```python
from build123d import *

# Parameters (mm, degrees)
SKETCH_2_W          = 24
SKETCH_2_H          = 28
EXTRUDE_1_DEPTH     = 22
SKETCH_3_W          = 20
SKETCH_3_H          = 24
CUT_EXTRUDE_1_DEPTH = 18
SKETCH_4_W          = 16
SKETCH_4_H          = 13
CUT_EXTRUDE_3_DEPTH = 26.768197453
SKETCH_6_W          = 20
SKETCH_6_H          = 24
CUT_EXTRUDE_4_DEPTH = 5
SKETCH_7_W          = 24
SKETCH_7_H          = 2
EXTRUDE_3_DEPTH     = 10
SKETCH_8_W          = 24
SKETCH_8_H          = 2
EXTRUDE_4_DEPTH     = 10
EXTRUDE_5_DEPTH     = 35
SKETCH_10_W         = 22
SKETCH_10_H         = 2
EXTRUDE_6_DEPTH     = 25
FILLET_2_R          = 5
SKETCH_11_W         = 7
SKETCH_11_H         = 10
CUT_EXTRUDE_5_DEPTH = 67.80007485
FILLET_4_R          = 2
SKETCH_12_W         = 20
SKETCH_12_H         = 13.5
EXTRUDE_7_DEPTH     = 8
RIB_1_REACH         = 64.944
SKETCH_14_W         = 22
SKETCH_14_H         = 5.5
EXTRUDE_8_DEPTH     = 45
FILLET_5_R          = 2


with BuildPart() as part:
    # ｽｹｯﾁ2 → ﾎﾞｽ - 押し出し1 (new body)
    with BuildSketch(Plane.XY):
        Rectangle(SKETCH_2_W, SKETCH_2_H)
    extrude(amount=EXTRUDE_1_DEPTH)

    # ｽｹｯﾁ3 → ｶｯﾄ - 押し出し1 (cut)
    with BuildSketch(Plane.XY.offset(22)):
        Rectangle(SKETCH_3_W, SKETCH_3_H)
    extrude(amount=-CUT_EXTRUDE_1_DEPTH, mode=Mode.SUBTRACT)

    # ｽｹｯﾁ4 → ｶｯﾄ - 押し出し3 (cut, through all)
    with BuildSketch(Plane.XY.offset(4)):
        with Locations((-4, 0)):
            Rectangle(SKETCH_4_W, SKETCH_4_H)
    extrude(amount=-CUT_EXTRUDE_3_DEPTH, mode=Mode.SUBTRACT)

    # ｽｹｯﾁ6 → ｶｯﾄ - 押し出し4 (cut)
    with BuildSketch(Plane.ZY.offset(12)):
        with Locations((12, 0)):
            Rectangle(SKETCH_6_W, SKETCH_6_H)
    extrude(amount=-CUT_EXTRUDE_4_DEPTH, mode=Mode.SUBTRACT)

    # ｽｹｯﾁ7 → ﾎﾞｽ - 押し出し3 (add)
    with BuildSketch(Plane.XZ.offset(14)):
        with Locations((0, 1)):
            Rectangle(SKETCH_7_W, SKETCH_7_H)
    extrude(amount=EXTRUDE_3_DEPTH)

    # ｽｹｯﾁ8 → ﾎﾞｽ - 押し出し4 (add)
    with BuildSketch(Plane(origin=(0, 14, 0), x_dir=(1, 0, 0), z_dir=(0, 1, 0))):
        with Locations((0, -1)):
            Rectangle(SKETCH_8_W, SKETCH_8_H)
    extrude(amount=EXTRUDE_4_DEPTH)

    # ｽｹｯﾁ9 → ﾎﾞｽ - 押し出し5 (add)
    with BuildSketch(Plane(origin=(0, 0, 0), x_dir=(-1, 0, 0), z_dir=(0, 0, -1))):
        Polygon((12, 17.5), (17, 17.5), (17, -17.5), (12, -17.5), (12, -12), (10, -12), (10, -19.5), (19, -19.5), (19, 19.5), (10, 19.5), (10, 12), (12, 12), align=None)
    extrude(amount=-EXTRUDE_5_DEPTH)

    # ｽｹｯﾁ10 → ﾎﾞｽ - 押し出し6 (add)
    with BuildSketch(Plane.XY.offset(22)):
        with Locations((1, 13)):
            Rectangle(SKETCH_10_W, SKETCH_10_H)
        with Locations((1, -13)):
            Rectangle(SKETCH_10_W, SKETCH_10_H)
    extrude(amount=EXTRUDE_6_DEPTH)

    # ﾌｨﾚｯﾄ2
    fillet_2_edges = [part.edges().sort_by_distance(p)[0] for p in [
        (11, 12, 22),
        (11, -12, 22),
    ]]
    fillet(fillet_2_edges, radius=FILLET_2_R)

    # ｽｹｯﾁ11 → ｶｯﾄ - 押し出し5 (cut, through all)
    with BuildSketch(Plane(origin=(0, 19.5, 0), x_dir=(1, 0, 0), z_dir=(0, 1, 0))):
        with Locations((-15.5, -5)):
            Rectangle(SKETCH_11_W, SKETCH_11_H)
    extrude(amount=-CUT_EXTRUDE_5_DEPTH, mode=Mode.SUBTRACT)

    # ﾌｨﾚｯﾄ4
    fillet_4_edges = [part.edges().sort_by_distance(p)[0] for p in [
        (-12, -18.5, 10),
        (-12, 18.5, 10),
    ]]
    fillet(fillet_4_edges, radius=FILLET_4_R)

    # ｽｹｯﾁ12 → ﾎﾞｽ - 押し出し7 (add)
    with BuildSketch(Plane(origin=(0, 0, 0), x_dir=(-1, 0, 0), z_dir=(0, 0, -1))):
        Polygon((-12, 24), (12, 24), (12, 6.5), (-4, 6.5), (-4, -6.5), (12, -6.5), (12, -24), (-12, -24), (-12, -6.5), (-12, 6.5), align=None)
        with Locations((0, -15.25)):
            Rectangle(SKETCH_12_W, SKETCH_12_H, mode=Mode.SUBTRACT)
        with Locations((0, 15.25)):
            Rectangle(SKETCH_12_W, SKETCH_12_H, mode=Mode.SUBTRACT)
    extrude(amount=EXTRUDE_7_DEPTH)

    # ｽｹｯﾁ13 walls → ﾘﾌﾞ1 (add, up to next)
    with BuildSketch(Plane(origin=(0, 0, -8), x_dir=(-1, 0, 0), z_dir=(0, 0, -1)), mode=Mode.PRIVATE) as rib_1_sk1:
        Polygon((-63.559720526, 56.946318504), (62.440774816, -28.104015852), (63.559720526, -26.446318504), (-62.440774816, 58.604015852), align=None)
    rib_1_tool1 = extrude(rib_1_sk1.sketch, amount=-RIB_1_REACH, mode=Mode.PRIVATE) - part.part
    # ｽｹｯﾁ13 walls → ﾘﾌﾞ1 (add, up to next)
    with BuildSketch(Plane(origin=(0, 0, -8), x_dir=(-1, 0, 0), z_dir=(0, 0, -1)), mode=Mode.PRIVATE) as rib_1_sk2:
        Polygon((-62.440774816, -28.104015852), (63.559720526, 56.946318504), (62.440774816, 58.604015852), (-63.559720526, -26.446318504), align=None)
    rib_1_tool2 = extrude(rib_1_sk2.sketch, amount=-RIB_1_REACH, mode=Mode.PRIVATE) - part.part
    # ｽｹｯﾁ13 walls → ﾘﾌﾞ1 (add, up to next)
    with BuildSketch(Plane(origin=(0, 0, -8), x_dir=(-1, 0, 0), z_dir=(0, 0, -1)), mode=Mode.PRIVATE) as rib_1_sk3:
        Polygon((-63.559720526, 26.446318504), (62.440774816, -58.604015852), (63.559720526, -56.946318504), (-62.440774816, 28.104015852), align=None)
    rib_1_tool3 = extrude(rib_1_sk3.sketch, amount=-RIB_1_REACH, mode=Mode.PRIVATE) - part.part
    # ｽｹｯﾁ13 walls → ﾘﾌﾞ1 (add, up to next)
    with BuildSketch(Plane(origin=(0, 0, -8), x_dir=(-1, 0, 0), z_dir=(0, 0, -1)), mode=Mode.PRIVATE) as rib_1_sk4:
        Polygon((-62.440774816, -58.604015852), (63.559720526, 26.446318504), (62.440774816, 28.104015852), (-63.559720526, -56.946318504), align=None)
    rib_1_tool4 = extrude(rib_1_sk4.sketch, amount=-RIB_1_REACH, mode=Mode.PRIVATE) - part.part
    add(rib_1_tool1.solids().sort_by_distance((0, 15.25, -8))[0])
    add(rib_1_tool2.solids().sort_by_distance((0, 15.25, -8))[0])
    add(rib_1_tool3.solids().sort_by_distance((0, -15.25, -8))[0])
    add(rib_1_tool4.solids().sort_by_distance((0, -15.25, -8))[0])

    # ｽｹｯﾁ14 → ﾎﾞｽ - 押し出し8 (add)
    with BuildSketch(Plane.XY.offset(2)):
        with Locations((1, 16.75)):
            Rectangle(SKETCH_14_W, SKETCH_14_H)
        with Locations((1, -16.75)):
            Rectangle(SKETCH_14_W, SKETCH_14_H)
    extrude(amount=EXTRUDE_8_DEPTH)

    # ﾌｨﾚｯﾄ5
    fillet_5_edges = [part.edges().sort_by_distance(p)[0] for p in [
        (0, -19.5, 2),
        (0, 19.5, 2),
        (-10, -15.75, 35),
        (-10, 15.75, 35),
    ]]
    fillet(fillet_5_edges, radius=FILLET_5_R)


solid = part.part
```
Work out the finished part from the listing and answer in its coordinate system (mm). A direction names the side the tool comes from. Round coordinates to 2 decimals unless told otherwise and drop trailing zeros. Loops run counter-clockwise (first coordinate to the right, second up) from the corner with the lowest first, then second, coordinate; pieces in that order, holes last. Notation, with made-up numbers: M 82.5,3.5 L 136.5,3.5 A9 ccw 136.5,7.5 Z; hole C -22,37.5 d7. An arc over 180 degrees is marked long. Use CSV: the item, a comma, the result in double quotes.
Q1. Each of these flat-tipped pins is pushed along its axis until it touches: pin 1 (2.5 mm diameter, centred on y = -15, z = -2, fed in from -X); pin 2 (10 mm diameter, centred on x = 4.5, z = 15, fed in from -Y); pin 3 (1 mm diameter, centred on y = -10, z = 3.5, fed in from -X); pin 4 (4 mm diameter, centred on x = -8, z = 3, fed in from -Y). Where does it stop, or does it pass through?
Determined:
pin 1,"x = -12"
pin 2,"y = -19.5"
pin 3,"x = -7"
pin 4,"y = -24"
Q2. The mould has two halves that part along X. Classify faces 6 (the flat face through (5, 0, 4)), 7 (the flat face through (-5.95, 12.44, -4.06)), 8 (the flat face through (4, 0, -2)): pulls with the +X half, pulls with the -X half, needs draft (parallel to the pull), parting line crosses it, or undercut.
Determined:
face 6,"needs draft"
face 7,"undercut"
face 8,"pulls with the -X half"
Q3. Consider L1, parallel to Y at x = -1, z = 30.5; L2, parallel to Y at x = -8.5, z = 1; L3, parallel to X at y = 10.5, z = 15.5. Determine where each line is inside the solid, lowest interval first.
Determined:
L1,"-19.5 to -12, 12 to 19.5"
L2,"-24 to -6.5, 6.5 to 24"
L3,"-19 to -17, 10 to 12"
Q4. Section C-C, the plane z = 12.5 is taken. Determine the outline of the cut face in (x, y), then the cut area to 3 significant figures.
Determined:
outline,"M -19,-19.5 L 12,-19.5 L 12,19.5 L -19,19.5 Z; hole M -17,-17.5 L -12,-17.5 L -12,-12 L 10,-12 L 10,12 L -12,12 L -12,17.5 L -17,17.5 Z"
area,"506 mm2"
Q5. Section B-B, the plane y = 2 is taken. Determine the outline of the cut face in (x, z), then the cut area to 3 significant figures.
Determined:
outline,"M -19,10 L -17,10 L -17,35 L -19,35 Z; M 4,-8 L 12,-8 L 12,22 L 10,22 L 10,4 L 4,4 Z"
area,"182 mm2"
Q6. A tool of negligible diameter and unlimited length cuts with its end or side. For faces 1 (the flat face through (0, 8.5, -4)), 2 (the flat face through (0, 12, 24)), 3 (the flat face through (-3, -19.5, 25)), 4 (the flat face through (-15, -17.5, 21)), 5 (the flat face through (-4, 6.5, -2)), from which of +Z, -Z, +X, -X, +Y, -Y can it reach the whole face along a straight path? Write none if from no direction.
Determined:
face 1,"-Z"
face 2,"+Z"
face 3,"+Z, +X, -X, -Y"
face 4,"+Z, -Z"
face 5,"+Z, -Z, -X"
Q7. Section A-A, the plane z = 41.5 is taken. Determine the outline of the cut face in (x, y), then the cut area to 3 significant figures.
Determined:
outline,"M -10,-19.5 L 12,-19.5 L 12,-12 L -10,-12 Z; M -10,12 L 12,12 L 12,19.5 L -10,19.5 Z"
area,"330 mm2"
